Autodesk Inventor part; units mm, degrees
ref_plane "Work Plane1" through (-21.15, -21.15, -31.5) normal (0, 0, -1) x (0, 1, 0)
ref_plane "YZ Plane" through (0, 0, 0) normal (1, 0, 0) x (0, 1, 0)
ref_plane "XZ Plane" through (0, 0, 0) normal (0, 1, 0) x (-1, 0, 0)
sketch "Sketch1" plane through (0, 0, 0) normal (0, 0, 1) x (1, 0, 0)
  line L0 (20.0607, 17.4322) -> (17.4322, 20.0607) construction
  arc A0 (17.4322, 20.0607) -> (16.3716, 20.5) centre (16.3716, 19) ccw construction
  line L1 (16.3716, 20.5) -> (-16.3716, 20.5) construction
  arc A1 (-16.3716, 20.5) -> (-17.4322, 20.0607) centre (-16.3716, 19) ccw construction
  line L2 (-17.4322, 20.0607) -> (-20.0607, 17.4322) construction
  arc A2 (-20.0607, 17.4322) -> (-20.5, 16.3716) centre (-19, 16.3716) ccw construction
  line L3 (-20.5, 16.3716) -> (-20.5, -16.3716) construction
  arc A3 (-20.5, -16.3716) -> (-20.0607, -17.4322) centre (-19, -16.3716) ccw construction
  line L4 (-20.0607, -17.4322) -> (-17.4322, -20.0607) construction
  arc A4 (-17.4322, -20.0607) -> (-16.3716, -20.5) centre (-16.3716, -19) ccw construction
  line L5 (-16.3716, -20.5) -> (16.3716, -20.5) construction
  arc A5 (16.3716, -20.5) -> (17.4322, -20.0607) centre (16.3716, -19) ccw construction
  line L6 (17.4322, -20.0607) -> (20.0607, -17.4322) construction
  arc A6 (20.0607, -17.4322) -> (20.5, -16.3716) centre (19, -16.3716) ccw construction
  line L7 (20.5, -16.3716) -> (20.5, 16.3716) construction
  arc A7 (20.5, 16.3716) -> (20.0607, 17.4322) centre (19, 16.3716) ccw construction
  circle A8 centre (0, 0) radius 16.5 construction
  circle A9 centre (15.5, 15.5) radius 1.55 construction
  circle A10 centre (15.5, -15.5) radius 1.55 construction
  circle A11 centre (-15.5, -15.5) radius 1.55 construction
  circle A12 centre (-15.5, 15.5) radius 1.55 construction
  line L8 (0, 0) -> (-20.3858, 0) construction
  line L9 (-20.3858, 0) -> (-20.3858, -20.3858) construction
  line L10 (-20.3858, -20.3858) -> (0, -20.3858) construction
  line L11 (0, -20.3858) -> (0, 0) construction
  line L12 (0, 0) -> (-20.3858, 0) construction
  line L13 (-20.3858, 0) -> (-20.3858, 20.3858) construction
  line L14 (-20.3858, 20.3858) -> (0, 20.3858) construction
  line L15 (0, 20.3858) -> (0, 0) construction
  line L16 (0, 0) -> (20.3858, 0) construction
  line L17 (20.3858, 0) -> (20.3858, 20.3858) construction
  line L18 (20.3858, 20.3858) -> (0, 20.3858) construction
  line L19 (0, 20.3858) -> (0, 0) construction
  line L20 (0, 0) -> (20.3858, 0) construction
  line L21 (20.3858, 0) -> (20.3858, -20.3858) construction
  line L22 (20.3858, -20.3858) -> (0, -20.3858) construction
  line L23 (0, -20.3858) -> (0, 0) construction
  line L24 (-20.3858, -20.3858) -> (20.3858, -20.3858)
  line L25 (20.3858, -20.3858) -> (20.3858, 20.3858)
  line L26 (20.3858, 20.3858) -> (-20.3858, 20.3858)
  line L27 (-20.3858, 20.3858) -> (-20.3858, -20.3858)
  line L28 (-21.15, -107.4) -> (-21.15, 107.4)
  line L29 (-21.15, 22.8858) -> (22.8858, 22.8858)
  line L30 (22.8858, 22.8858) -> (22.8858, -22.8858)
  line L31 (22.8858, -22.8858) -> (-21.15, -22.8858)
  point P0 (0, 0)
  dimension "d0" = 2.5
ref_plane "Work Plane1" through (-21.15, -21.15, -31.5) normal (0, 0, -1) x (0, 1, 0)
extrude "Extrusion1" add sketch "Sketch1" against normal up to surface (31.5 mm away)
ref_plane "Work Plane2" through (-21.15, -10, -125) normal (1, 0, 0) x (0, 0, 1)
sketch "Sketch2" plane through (-21.15, -10, -125) normal (1, 0, 0) x (0, 0, 1)
  line L0 (125, 12.8858) -> (125, -32.8858)
  line L1 (93.5, 12.8858) -> (93.5, -32.8858)
  line L2 (125, -32.8858) -> (93.5, -32.8858)
  line L3 (125, 12.8858) -> (125, -32.8858)
  line L4 (125, 12.8858) -> (93.5, 12.8858)
  line L5 (125, -10) -> (93.5, -10) construction
  line L6 (109.25, 12.8858) -> (109.25, -32.8858) construction
  line L7 (109.25, -32.8858) -> (119.25, -32.8858) construction
  line L8 (119.25, -32.8858) -> (119.25, -42.8858)
  line L9 (119.25, -42.8858) -> (109.25, -42.8858)
  line L10 (109.25, -42.8858) -> (109.25, -32.8858) construction
  line L11 (109.25, -42.8858) -> (99.25, -42.8858)
  line L12 (99.25, -42.8858) -> (99.25, -32.8858)
  line L13 (99.25, -32.8858) -> (109.25, -32.8858) construction
  line L14 (109.25, -32.8858) -> (109.25, -42.8858) construction
  line L15 (125, 12.8858) -> (93.5, 12.8858)
  line L16 (119.25, 12.8858) -> (119.25, 22.8858)
  line L17 (119.25, 22.8858) -> (109.25, 22.8858)
  line L18 (109.25, 22.8858) -> (99.25, 22.8858)
  line L19 (99.25, 22.8858) -> (99.25, 12.8858)
  dimension "d3" = 10
  dimension "d4" = 10
  dimension "d5" = 10
  dimension "d6" = 10
extrude "Extrusion2" add sketch "Sketch2" along normal blind 5 contours L4 L19 L18 L17 L16 | L8 L9 L11 L12 L2
sketch "Sketch3" plane through (0, 0, 0) normal (0, 0, 1) x (1, 0, 0)
  line L0 (22.8858, 22.8858) -> (-21.15, 22.8858)
  line L1 (-21.15, 22.8858) -> (-21.15, -22.8858)
  line L2 (22.8858, 22.8858) -> (-21.15, 22.8858)
  line L3 (-21.15, 22.8858) -> (-21.15, -22.8858)
  line L4 (-21.15, -22.8858) -> (22.8858, -22.8858)
  line L5 (22.8858, -22.8858) -> (22.8858, 22.8858)
  circle A0 centre (-15.5, 15.5) radius 1.25
  circle A1 centre (15.5, 15.5) radius 1.25
  circle A2 centre (-15.5, -15.5) radius 1.25
  circle A3 centre (15.5, -15.5) radius 1.25
  circle A4 centre (0, 0) radius 11
  point P0 (0, 0)
extrude "Extrusion3" add sketch "Sketch3" along normal blind 1
fillet "Fillet1" radius 2 10 edges at (-18.65, 22.8858, -25.75) (-18.65, 32.8858, -25.75) (-18.65, 32.8858, -5.75) (-18.65, 22.8858, -5.75) (-18.65, -22.8858, -25.75) (-18.65, -32.8858, -25.75) (-18.65, -32.8858, -5.75) (-18.65, -22.8858, -5.75) (-16.15, -22.8858, -15.75) (-16.15, 22.8858, -15.75)
sketch "Sketch4" plane through (-16.15, -10, -125) normal (1, 0, 0) x (0, 0, -1)
  arc A0 (-117.25, 42.8858) -> (-119.25, 40.8858) centre (-117.25, 40.8858) ccw
  line L0 (-119.25, 40.8858) -> (-119.25, 34.8858)
  line L1 (-99.25, 34.8858) -> (-119.25, 34.8858)
  line L2 (-99.25, 34.8858) -> (-99.25, 40.8858)
  arc A1 (-99.25, 40.8858) -> (-101.25, 42.8858) centre (-101.25, 40.8858) ccw
  line L3 (-101.25, 42.8858) -> (-117.25, 42.8858)
  arc A2 (-119.25, -20.8858) -> (-117.25, -22.8858) centre (-117.25, -20.8858) ccw
  line L4 (-117.25, -22.8858) -> (-101.25, -22.8858)
  arc A3 (-101.25, -22.8858) -> (-99.25, -20.8858) centre (-101.25, -20.8858) ccw
  line L5 (-99.25, -20.8858) -> (-99.25, -14.8858)
  line L6 (-119.25, -14.8858) -> (-99.25, -14.8858)
  line L7 (-119.25, -14.8858) -> (-119.25, -20.8858)
  circle A4 centre (-109.25, 38.7448) radius 2.5
  line L8 (-215.88, 9.0017) -> (215.88, 9.0017) construction
  line L9 (-126, 32.8858) -> (-126, -12.8858) construction
  line L10 (-126, 10) -> (-93.5, 10) construction
  line L11 (-93.5, 32.8858) -> (-93.5, -12.8858) construction
  circle A5 centre (-109.25, -18.7448) radius 2.5
  point P0 (-125, 10)
  dimension "d12" = 5
extrude "Extrusion4" cut sketch "Sketch4" against normal up to surface (5 mm away) contours A4 | A5
properties part number "Nema17WheelMotorMount"
Design review of the part built by this model. Coordinates are the model's own, in mm. A direction names the side the tool comes from. Round coordinates to 2 decimals unless told otherwise and drop trailing zeros. Write each loop counter-clockwise with the first axis right and the second up, starting at its lowest first coordinate (ties: lowest second). Pieces come first, ordered by that corner, then holes. Notation, with made-up numbers: (31, 59) -> (69, 59) arc R15 ccw to (69, 66) -> close; hole circle Ø8 at (1, -38.75). An arc over 180 degrees is marked (long way). One line per item, written item: value. Start each with the question number.
Q1. Add section D-D (x = 15.5). Give the boundary of the cut face in (y, z).
Q2. Add section C-C (y = 0). Give the boundary of the cut face in (x, z).
Q3. To check wall thickness, follow probe 1 along Y at (x, z) = (15.5, 0.65); probe 2 along Y at (x, z) = (0, -6); probe 3 along X at (y, z) = (4.5, -3.5). State the ranges of each line that lie inside material, in increasing order.
Q4. The part is to be moulded in two halves that separate along X. For faces 4 (the face through (-19, 28, -25.75)), 5 (the face through (-16.15, 31.5, -15.9)), 6 (the face through (9, 9, 0)), say which applies: pulls with the +X half, pulls with the -X half, needs draft (parallel to the pull), parting line crosses it, or undercut.
Q5. Add section B-B (z = -15.75). Give the boundary of the cut face in (x, y).
Q6. Add section A-A (x = 0). Give the boundary of the cut face in (y, z).
Q7. Insertion check: P1, Ø4, axis at x = -19, y = -29, coming from the +Z side; P2, Ø1.5, axis at x = -18.5, y = -27, coming from the -Z side; P3, Ø4, axis at y = -30, z = -20.5, coming from the +X side. Each pin has a flat end and moves straight along its axis. Give the tip position at first contact, or say it passes through.
Q8. Tool access review of faces 1 (the face through (-21.15, 0, -15)), 2 (the face through (0, -20.386, -16)), 3 (the face through (-19, 28, -5.75)): name each direction out of +Z, -Z, +X, -X, +Y, -Y from which nothing blocks a thin tool from reaching the whole face with its end or side.
Response:
1. outline: (-22.89, -31.5) -> (-20.39, -31.5) -> (-20.39, 0) -> (-16.75, 0) -> (-16.75, 1) -> (-22.89, 1) -> close; (-14.25, 0) -> (14.25, 0) -> (14.25, 1) -> (-14.25, 1) -> close; (16.75, 0) -> (20.39, 0) -> (20.39, -31.5) -> (22.89, -31.5) -> (22.89, 1) -> (16.75, 1) -> close
2. outline: (-21.15, -31.5) -> (-20.39, -31.5) -> (-20.39, 0) -> (-11, 0) -> (-11, 1) -> (-21.15, 1) -> close; (11, 0) -> (20.39, 0) -> (20.39, -31.5) -> (22.89, -31.5) -> (22.89, 1) -> (11, 1) -> close
3. probe 1: y = -22.89 to -16.75, -14.25 to 14.25, 16.75 to 22.89
3. probe 2: y = -22.89 to -20.39, 20.39 to 22.89
3. probe 3: x = -21.15 to -20.39, 20.39 to 22.89
4. face 4: needs draft
4. face 5: pulls with the +X half
4. face 6: undercut
5. outline: (-21.15, -32.89) -> (-16.15, -32.89) -> (-16.15, -31.24) -> (-21.15, -31.24) -> close; (-21.15, -26.24) -> (-16.15, -26.24) -> (-16.15, -24.89) arc R2 cw to (-14.15, -22.89) -> (22.89, -22.89) -> (22.89, 22.89) -> (-14.15, 22.89) arc R2 cw to (-16.15, 24.89) -> (-16.15, 26.24) -> (-21.15, 26.24) -> close; (-21.15, 31.24) -> (-16.15, 31.24) -> (-16.15, 32.89) -> (-21.15, 32.89) -> close; hole (-20.39, -20.39) -> (20.39, -20.39) -> (20.39, 20.39) -> (-20.39, 20.39) -> close
6. outline: (-22.89, -31.5) -> (-20.39, -31.5) -> (-20.39, 0) -> (-11, 0) -> (-11, 1) -> (-22.89, 1) -> close; (11, 0) -> (20.39, 0) -> (20.39, -31.5) -> (22.89, -31.5) -> (22.89, 1) -> (11, 1) -> close
7. P1: stops at z = -5.75
7. P2: stops at z = -25.75
7. P3: stops at x = -16.15
8. face 1: +Z, -Z, -X, +Y, -Y
8. face 2: -Z
8. face 3: +Z, +X, -X, +Y
